Can you work these out from the model? Positions are in its coordinate system, mm. A direction names the side the tool comes from. Round coordinates to 2 decimals unless told otherwise and drop trailing zeros. Write each loop counter-clockwise with the first axis right and the second up, starting at its lowest first coordinate (ties: lowest second). Pieces come first, ordered by that corner, then holes.
Q1. For faces 1 (the flat face through (5, -50.8, 4)), 2 (the flat face through (6.35, 12, 13)), 3 (the cylindrical face through (0.133, -86.34, 16.716)), which set-ups out of +Z, -Z, +X, -X, +Y, -Y let a thin tool reach every point of the face, with its end or its side?
Q2. If we section it at B-B (x = 0): Please give me the cut outline in (y, z) (1 decimal).
Q3. Please list where these lines run through material, in increasing order: line 1 along Z through (x, y) = (-8.75, 38.1); line 2 along X through (y, z) = (24.5, 12); line 3 along Y through (x, z) = (-2.5, 12.7).
Q4. We'd pull the mould along X, two halves only. Please class faces 4 (the flat face through (9, 50.8, 13)), 5 (the flat face through (12.7, -1, 13)), 6 (the flat face through (0, -25.4, 13)): +X half, -X half, draft (parallel to the pull), parting line (faces both ways), or undercut.
Q5. I'm going to push flat-ended pins straight in: pin 1 Ø2 at (x, y) = (-2.5, -47.5) entering from -Z; pin 2 Ø4 at (y, z) = (-308.5, 10) entering from +X; pin 3 Ø4 at (x, z) = (-1.5, 14) entering from +Y. Where does each tip first touch, or does it pass through?
Q6. If we section it at A-A (y = 38.1): Please give me the cut outline in (x, z).
from build123d import *

# Parameters (mm, degrees)
F0_W     = 25.4
F0_H     = 101.6
F1_DEPTH = 25.4
F2_W     = 12.7
F2_H     = 101.6
F3_DEPTH = 25.401
F4_R     = 6.35
F5_DEPTH = 25.401
F6_R     = 9.525
F7_DEPTH = 304.8
F8_R     = 4.7625
F9_DEPTH = 25.401


with BuildPart() as f1:
    # F0 (on Top) → F1 (new body)
    with BuildSketch(Plane.XY):
        Rectangle(F0_W, F0_H)
    extrude(amount=F1_DEPTH)

    # F2 (on face) → F3 (cut, through all)
    with BuildSketch(Plane.XY.offset(25.4)):
        with Locations((0, 25.4)):
            Rectangle(F2_W, F2_H)
    extrude(amount=-F3_DEPTH, mode=Mode.SUBTRACT)

    # F4 (on face) → F5 (cut, through all)
    with BuildSketch(Plane.YZ.offset(12.7)):
        with Locations((38.1, 12.7)):
            Circle(F4_R)
    extrude(amount=-F5_DEPTH, mode=Mode.SUBTRACT)

    # F6 (on face) → F7 (join)
    with BuildSketch(Plane.XZ.offset(50.8)):
        with Locations((0, 12.7)):
            Circle(F6_R)
    extrude(amount=F7_DEPTH)

    # F8 (on face) → F9 (cut, through all)
    with BuildSketch(Plane.YZ.offset(12.7)):
        with Locations((-88.9, 12.7)):
            Circle(F8_R)
    extrude(amount=-F9_DEPTH, mode=Mode.SUBTRACT)


solid = f1.part
A:
1. face 1: -Y
1. face 2: +Z, -Z, +Y
1. face 3: +X, -X
2. outline: (-355.6, 3.2) - (-50.8, 3.2) - (-50.8, 0) - (-25.4, 0) - (-25.4, 25.4) - (-50.8, 25.4) - (-50.8, 22.2) - (-355.6, 22.2) - close; hole circle Ø9.5 at (-88.9, 12.7)
3. line 1: z = 0 to 6.35, 19.05 to 25.4
3. line 2: x = -12.7 to -6.35, 6.35 to 12.7
3. line 3: y = -355.6 to -93.66, -84.14 to -25.4
4. face 4: draft
4. face 5: +X half
4. face 6: undercut
5. pin 1: stops at z = 0
5. pin 2: stops at x = 9.5
5. pin 3: stops at y = -25.4
6. outline: (-12.7, 0) - (-6.35, 0) - (-6.35, 6.35) - (-12.7, 6.35) - close; (-12.7, 19.05) - (-6.35, 19.05) - (-6.35, 25.4) - (-12.7, 25.4) - close; (6.35, 0) - (12.7, 0) - (12.7, 6.35) - (6.35, 6.35) - close; (6.35, 19.05) - (12.7, 19.05) - (12.7, 25.4) - (6.35, 25.4) - close
